Design review of the part built by this model. Coordinates are the model's own, in mm. A direction names the side the tool comes from. Coordinates: 2 decimals unless noted, no trailing zeros. Loops run counter-clockwise (first coordinate to the right, second up) from the corner with the lowest first, then second, coordinate; pieces in that order, holes last. Notation, with made-up numbers: M 51,39.5 L 67,39.5 A8 cw 67,53.5 Z; hole C -2.75,61 d1. An arc over 180 degrees is marked long. Put each result on its own line as item: value. Start each with the question number.
(1) Take a section at A-A, the plane x = 0. Give the boundary of the cut face in (y, z).
(2) For faces 1 (the cylindrical face through (5.598, 42.634, 1.014)), 2 (the flat face through (-34, -23, 5)), list the 3-axis set-ups (+Z, -Z, +X, -X, +Y, -Y) from which the entire face can be reached by the end or side of a thin tool; tool diameter is ignored.
(3) The part is to be moulded in two halves that separate along X. For faces 3 (the flat face through (-13, -38, 2)), 4 (the flat face through (-0.7, 43.3, 0)), 5 (the cylindrical face through (-8.67, -39.05, 3.48)), 6 (the flat face through (49.5, -1, 2)), say which applies: +X half, -X half, draft (parallel to the pull), parting line (faces both ways), or undercut.
(4) Take a section at C-C, the plane z = 3.65. Give the boundary of the cut face in (x, y).
(5) For probe 1 along X at (y, z) = (0, 0.85); probe 2 along X at (y, z) = (0, 3.8), list the stretches that pass through material, from the lowest coordinate up. Write a range as [from, to].
(6) Clearance check with a flat-ended pin moving along its axis: pin 1 (3 mm diameter, centred on x = 12, y = -38.5, fed in from -Z). State where the tip first meets the part, or that it passes through.
```python
from build123d import *

# Parameters (mm, degrees)
SKETCH1_W               = 99
SKETCH1_H               = 99
SKETCH1_R               = 40
BOSS_EXTRUDE1_DEPTH     = 5
CUT_EXTRUDE1_DEPTH      = 71.1819065
CUT_EXTRUDE1_DEPTH_BACK = 2
SKETCH2_R               = 43
CHAMFER1_SIZE           = 1


with BuildPart() as part:
    # Sketch1 → Boss-Extrude1 (new body)
    with BuildSketch(Plane(origin=(0, 0, 0), x_dir=(0, 1, 0), z_dir=(0, 0, 1))):
        Rectangle(SKETCH1_W, SKETCH1_H)
        with Locations(Location((0, 0, 0), (0, 0, 270))):
            Circle(SKETCH1_R, mode=Mode.SUBTRACT)
    extrude(amount=BOSS_EXTRUDE1_DEPTH)

    # Sketch2 → Cut-Extrude1 (cut, two sides: drawn at the far end of the back side and taken through both)
    with BuildSketch(Plane(origin=(0, 0, 0), x_dir=(1, 0, 0), z_dir=(0, 0, -1)).offset(-CUT_EXTRUDE1_DEPTH_BACK)):
        with Locations(Location((0, 0, 0), (0, 0, 180))):
            Circle(SKETCH2_R)
    extrude(amount=CUT_EXTRUDE1_DEPTH + CUT_EXTRUDE1_DEPTH_BACK, mode=Mode.SUBTRACT)

    # Chamfer1
    chamfer1_edges = [part.edges().sort_by_distance(p)[0] for p in [
        (-49.5, -49.5, 2.5),
        (-49.5, 49.5, 2.5),
        (49.5, 49.5, 2.5),
        (49.5, -49.5, 2.5),
    ]]
    chamfer(chamfer1_edges, length=CHAMFER1_SIZE)


solid = part.part
```
Computed values:
1. outline: M -49.5,0 L -43,0 L -43,2 L -40,2 L -40,5 L -49.5,5 Z; M 40,2 L 43,2 L 43,0 L 49.5,0 L 49.5,5 L 40,5 Z
2. face 1: -Z
2. face 2: +Z, +X, -X, +Y, -Y
3. face 3: undercut
3. face 4: draft
3. face 5: undercut
3. face 6: +X half
4. outline: M -49.5,-48.5 L -48.5,-49.5 L 48.5,-49.5 L 49.5,-48.5 L 49.5,48.5 L 48.5,49.5 L -48.5,49.5 L -49.5,48.5 Z; hole C 0,0 d80
5. probe 1: x = [-49.5, -43], [43, 49.5]
5. probe 2: x = [-49.5, -40], [40, 49.5]
6. pin 1: stops at z = 2
